For this review, use the dimensioned drawing (mm, ordinates from the lowest corner) and the shaded views. A direction names the side the tool comes from. Give positions to 0.01 mm unless a question says otherwise; leave off trailing zeros. Loops run counter-clockwise (first coordinate to the right, second up) from the corner with the lowest first, then second, coordinate; pieces in that order, holes last. Notation, with made-up numbers: (75.25, 23.5) -> (86.25, 23.5) arc R26 cw to (86.25, 53.5) -> close; hole circle Ø8 at (85.5, 75). An arc over 180 degrees is marked (long way). Use a Markdown table: item, result. Add a question column.
1. Add section B-B (x = 48.1). State the section outline as (y, z) points.
2. For pin 1 Ø4 at (y, z) = (11, 10) entering from -X; pin 2 Ø2.5 at (x, z) = (1.5, 10.5) entering from +Y; pin 3 Ø7 at (x, z) = (28, 4.5) entering from -Y; pin 4 Ø1.8 at (x, z) = (48.1, 4) entering from +Y, all flat-tipped, find the tip position at first contact; note any pin that passes through.
3. Add section C-C (z = 4). State the section outline as (x, y) points, and give its area (3 significant figures).
4. For the marked faces 1, 2 and 3, list the 3-axis set-ups (+Z, -Z, +X, -X, +Y, -Y) from which the entire face can be reached by the end or side of a thin tool; tool diameter is ignored.
5. Add section D-D (z = 8.5). State the section outline as (x, y) points, and give its area (3 significant figures).
6. Draft analysis for pull direction X (two halves, no side actions). For the marked faces 4, 5 and 6, state which applies: pulls with the +X half, pulls with the -X half, needs draft (parallel to the pull), parting line crosses it, or undercut.
7. To check wall thickness, follow line 1 (X direction, y = 0.85, z = 4); line 2 (Z direction, x = 48.1, y = 1.3); line 3 (X direction, y = 16.75, z = 4.5). State the ranges of each line that lie inside material, in increasing order.
8. Add section A-A (y = 8.75). State the section outline as (x, z) points.
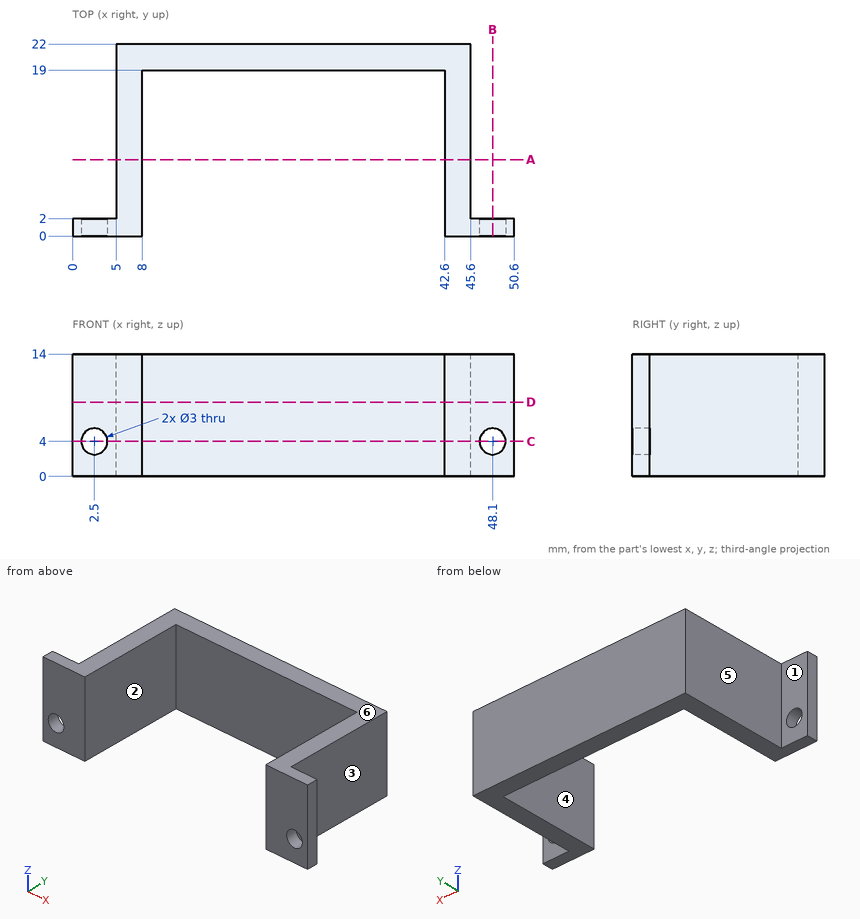
Taken from the geometry:
| question | item | result |
|---|---|---|
| 1 | outline | (0, 0) -> (2, 0) -> (2, 2.5) -> (0, 2.5) -> close; (0, 5.5) -> (2, 5.5) -> (2, 14) -> (0, 14) -> close |
| 2 | pin 1 | stops at x = 5 |
| 2 | pin 2 | stops at y = 2 |
| 2 | pin 3 | stops at y = 19 |
| 2 | pin 4 | passes through |
| 3 | outline | (0, 0) -> (1, 0) -> (1, 2) -> (0, 2) -> close; (4, 0) -> (8, 0) -> (8, 19) -> (42.6, 19) -> (42.6, 0) -> (46.6, 0) -> (46.6, 2) -> (45.6, 2) -> (45.6, 22) -> (5, 22) -> (5, 2) -> (4, 2) -> close; (49.6, 0) -> (50.6, 0) -> (50.6, 2) -> (49.6, 2) -> close |
| 3 | area | 244 mm^2 |
| 4 | face 1 | +Z, -Z, -X, +Y |
| 4 | face 2 | +Z, -Z, -Y |
| 4 | face 3 | +Z, -Z, +X, +Y |
| 5 | outline | (0, 0) -> (8, 0) -> (8, 19) -> (42.6, 19) -> (42.6, 0) -> (50.6, 0) -> (50.6, 2) -> (45.6, 2) -> (45.6, 22) -> (5, 22) -> (5, 2) -> (0, 2) -> close |
| 5 | area | 256 mm^2 |
| 6 | face 4 | undercut |
| 6 | face 5 | pulls with the -X half |
| 6 | face 6 | needs draft |
| 7 | line 1 | x = 0 to 1, 4 to 8, 42.6 to 46.6, 49.6 to 50.6 |
| 7 | line 2 | z = 0 to 2.5, 5.5 to 14 |
| 7 | line 3 | x = 5 to 8, 42.6 to 45.6 |
| 8 | outline | (5, 0) -> (8, 0) -> (8, 14) -> (5, 14) -> close; (42.6, 0) -> (45.6, 0) -> (45.6, 14) -> (42.6, 14) -> close |
